The drawing under review shows one solid part. Ordinate dimensions are in mm from its lowest x, y, z. Round coordinates to 2 decimals unless told otherwise and drop trailing zeros. Write each loop counter-clockwise with the first axis right and the second up, starting at its lowest first coordinate (ties: lowest second). Pieces come first, ordered by that corner, then holes. Notation, with made-up numbers: (72, -28) -> (82, -28) arc R6 cw to (82, -18) -> close; hole circle Ø10 at (40.5, -38). An arc over 180 degrees is marked (long way). Answer in a Markdown table with one row per item.
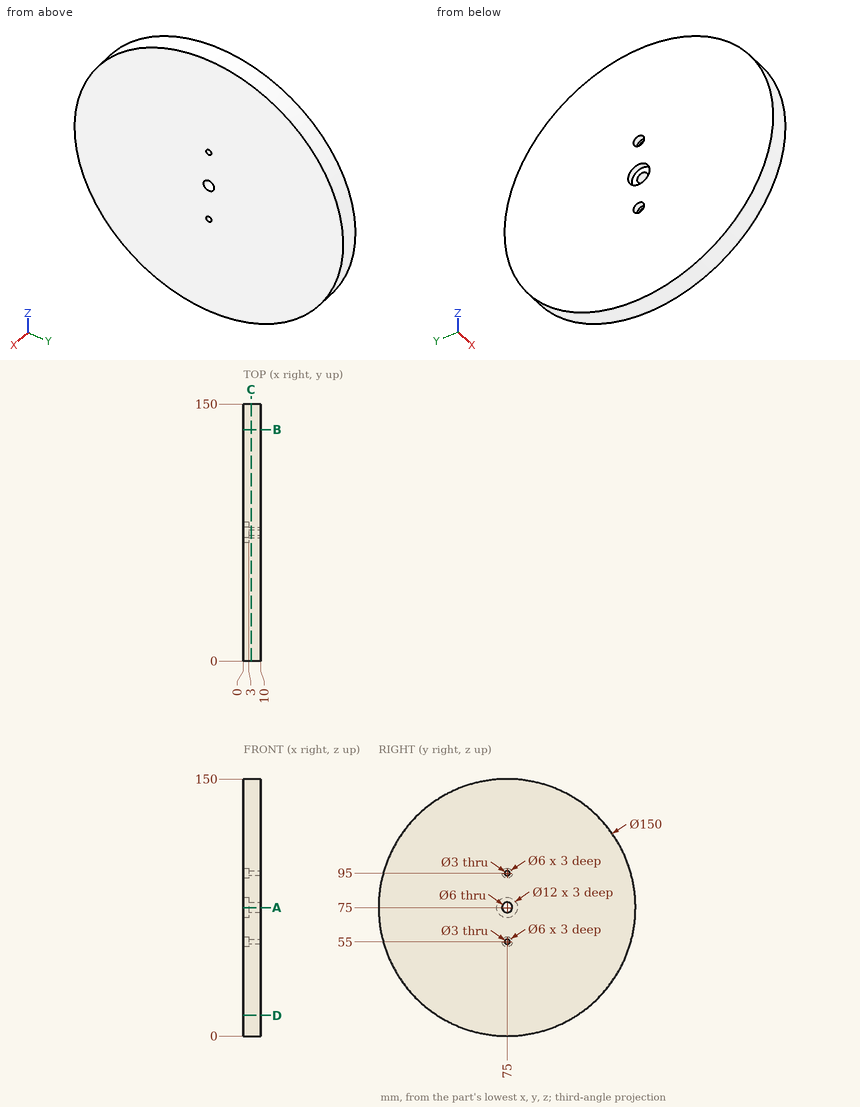
1) Consider section D-D on z = 12. State the section outline as (x, y) points.
Solved:
| item | result |
|---|---|
| outline | (0, 34.31) -> (10, 34.31) -> (10, 115.69) -> (0, 115.69) -> close |
2) Consider section B-B on y = 135. State the section outline as (x, z) points, then the cut area to 3 significant figures.
Solved:
| item | result |
|---|---|
| outline | (0, 30) -> (10, 30) -> (10, 120) -> (0, 120) -> close |
| area | 900 mm² |
3) Consider section C-C on x = 4.5. State the section outline as (y, z) points.
Solved:
| item | result |
|---|---|
| outline | circle Ø150 at (75, 75); hole circle Ø6 at (75, 75); hole circle Ø3 at (75, 55); hole circle Ø3 at (75, 95) |
4) Consider section A-A on z = 75. State the section outline as (x, y) points, then the cut area to 3 significant figures.
Solved:
| item | result |
|---|---|
| outline | (0, 0) -> (10, 0) -> (10, 72) -> (3, 72) -> (3, 69) -> (0, 69) -> close; (0, 81) -> (3, 81) -> (3, 78) -> (10, 78) -> (10, 150) -> (0, 150) -> close |
| area | 1,420 mm² |
5) Clearance check with flat-ended pins moving along their axes: pin 1 Ø2 at (x, z) = (6, 77.5) entering from +Y (3 decimals); pin 2 Ø5 at (x, z) = (6, 39) entering from -Y; pin 3 Ø4 at (x, z) = (7, 80.5) entering from +Y. State where each tip first meets the part, or that it passes through.
Solved:
| item | result |
|---|---|
| pin 1 | y = 149.985 |
| pin 2 | y = 7.9 |
| pin 3 | y = 149.92 |
6) For line 1 (Y direction, x = 0.8, z = 75); line 2 (Y direction, x = 7.75, z = 75); line 3 (Z direction, x = 2.25, y = 77), list the stretches that pass through material, from the lowest coordinate up. Write a range as [from, to].
Solved:
| item | result |
|---|---|
| line 1 | [0, 69], [81, 150] |
| line 2 | [0, 72], [78, 150] |
| line 3 | [0.03, 52.76], [57.24, 69.34], [80.66, 92.76], [97.24, 149.97] |
